Model file for the job. Use its own axes, mm. A direction names the side the tool comes from. Round coordinates to 2 decimals unless told otherwise and drop trailing zeros. Loops run counter-clockwise (first coordinate to the right, second up) from the corner with the lowest first, then second, coordinate; pieces in that order, holes last. Notation, with made-up numbers: M 78,15 L 137,15 A19 ccw 137,48 Z; hole C -17.5,-13 d11. An arc over 180 degrees is marked long. Use a Markdown table: item, result. Add a question column.
Item 1: Saw through at B-B on y = -10. Write the cut outline in (x, z).
Item 2: Saw through at D-D on z = 28. Write the cut outline in (x, y), then the cut area to 3 significant figures.
Item 3: Two-plate mould, pull along X, no slides. Class faces 1 (the flat face through (-2, -6, -35)), 2 (the flat face through (-10, -12.5, 8)), 3 (the cylindrical face through (-1.73, 7.81, -28.92)): +X half, -X half, draft (parallel to the pull), parting line (faces both ways), or undercut.
Item 4: Pin check, flat tips, straight feed: P1, Ø13, axis at x = -13.5, z = 17, coming from the -Y side; P2, Ø10, axis at y = -4, z = -30, coming from the -X side; P3, Ø1, axis at y = -7, z = -27, coming from the +X side; P4, Ø2, axis at y = -6, z = -30, coming from the -X side (3 decimals). Stop position of each tip, or through.
Item 5: Saw through at A-A on z = 0. Write the cut outline in (x, y).
Item 6: Wall check: L1, parallel to X at y = -4.25, z = 0; L2, parallel to Y at x = 14.5, z = 19; L3, parallel to Z at x = -20, y = -0.5. Give the ranges that are in metal, low to high. Write a range as from..to.
Item 7: Tool access for faces 4 (the cylindrical face through (6, 0, -40)), 5 (the flat face through (-19, -11, -19)), 6 (the flat face through (-19, 11, 18)): list every direction of +Z, -Z, +X, -X, +Y, -Y with a clear straight run to the whole face (end or side of a thin tool).
Item 8: Saw through at C-C on y = 0. Write the cut outline in (x, z), then the cut area to 3 significant figures.
```python
from build123d import *

# Parameters (mm, degrees)
SKETCH1_W           = 46
SKETCH1_H           = 46
BOSS_EXTRUDE1_DEPTH = 11
SKETCH2_R           = 19
BOSS_EXTRUDE2_DEPTH = 4.5
FILLET1_R           = 5
SKETCH3_R           = 16
CUT_EXTRUDE1_DEPTH  = 3
SKETCH4_R           = 12.5
CUT_EXTRUDE2_DEPTH  = 41.127920628
MIRROR1_START       = -12.5
MIRROR1_OUTLINE_R   = 16
MIRROR1_DEPTH       = 23.5
MIRROR1_START_2     = -15.5
MIRROR1_2_OUTLINE_W = 46
MIRROR1_2_OUTLINE_H = 46
MIRROR1_2_OUTLINE_R = 16
MIRROR1_2_DEPTH     = 4.5
SKETCH5_R           = 12.5
CUT_EXTRUDE3_DEPTH  = 42.955333564
SKETCH6_R           = 8
BOSS_EXTRUDE3_DEPTH = 12
SKETCH7_R           = 6
BOSS_EXTRUDE4_DEPTH = 10


with BuildPart() as part:
    # Sketch1 → Boss-Extrude1 (new, symmetric)
    with BuildSketch(Plane(origin=(0, 0, 0), x_dir=(1, 0, 0), z_dir=(0, 1, 0))):
        Rectangle(SKETCH1_W, SKETCH1_H)
    extrude(amount=BOSS_EXTRUDE1_DEPTH, both=True)

    # Sketch2 → Boss-Extrude2 (add)
    with BuildSketch(Plane(origin=(0, 11, 0), x_dir=(1, 0, 0), z_dir=(0, 1, 0))):
        with Locations(Location((0, 0, 0), (0, 0, 270))):
            Circle(SKETCH2_R)
    extrude(amount=BOSS_EXTRUDE2_DEPTH)

    # Fillet1
    # the kernel refuses this fillet: 5 mm, written as the material it adds along each edge
    with BuildSketch(Plane(origin=(0, 11, 0), x_dir=(0, 0, 1), z_dir=(-1, 0, 0))) as fillet1_piece_1_section:
        with BuildLine():
            CenterArc((23.974937186, 5), FILLET1_R, 185.739170477, 84.260829523)
            Line((19, 4.5), (19, 0))
            Line((19, 0), (23.974937186, 0))
        make_face()
    fillet1_piece_1 = revolve(axis=Axis((0, 11, 0), (0, 1, 0)), mode=Mode.PRIVATE)
    fillet1_piece_1 = split(fillet1_piece_1, bisect_by=Plane(origin=(0, 11, 23), z_dir=(0, 0, -1)), keep=Keep.TOP, mode=Mode.PRIVATE)
    fillet1_piece_1 = split(fillet1_piece_1, bisect_by=Plane(origin=(23, 11, 0), z_dir=(-1, 0, 0)), keep=Keep.TOP, mode=Mode.PRIVATE)
    fillet1_piece_1 = split(fillet1_piece_1, bisect_by=Plane(origin=(-23, 11, 0), z_dir=(1, 0, 0)), keep=Keep.TOP, mode=Mode.PRIVATE)
    fillet1_piece_1 = split(fillet1_piece_1, bisect_by=Plane(origin=(0, 11, -23), z_dir=(0, 0, 1)), keep=Keep.TOP, mode=Mode.PRIVATE)
    add(fillet1_piece_1)

    # Sketch3 → Cut-Extrude1 (cut)
    with BuildSketch(Plane(origin=(0, 15.5, 0), x_dir=(1, 0, 0), z_dir=(0, 1, 0))):
        with Locations(Location((0, 0, 0), (0, 0, 270))):
            Circle(SKETCH3_R)
    extrude(amount=-CUT_EXTRUDE1_DEPTH, mode=Mode.SUBTRACT)

    # Sketch4 → Cut-Extrude2 (cut, through all)
    with BuildSketch(Plane(origin=(0, 12.5, 0), x_dir=(1, 0, 0), z_dir=(0, 1, 0))):
        with Locations(Location((0, 0, 0), (0, 0, 270))):
            Circle(SKETCH4_R)
    extrude(amount=-CUT_EXTRUDE2_DEPTH, mode=Mode.SUBTRACT)

    # Mirror1: read off the stored shape, not the designer's step
    # Mirror1 outline → Mirror1 (add)
    with BuildSketch(Plane(origin=(0, 0, 0), x_dir=(1, 0, 0), z_dir=(0, 1, 0)).offset(MIRROR1_START)):
        Circle(MIRROR1_OUTLINE_R)
    extrude(amount=MIRROR1_DEPTH)

    # Mirror1 2 outline → Mirror1 2 (add)
    with BuildSketch(Plane(origin=(0, 0, 0), x_dir=(1, 0, 0), z_dir=(0, 1, 0)).offset(MIRROR1_START_2)):
        Rectangle(MIRROR1_2_OUTLINE_W, MIRROR1_2_OUTLINE_H)
        Circle(MIRROR1_2_OUTLINE_R, mode=Mode.SUBTRACT)
    extrude(amount=MIRROR1_2_DEPTH)

    # Mirror1 3 outline → Mirror1 3 (revolve, cut)
    with BuildSketch(Plane.XY):
        with BuildLine():
            Line((32.526911935, -11), (23.974937186, -11))
            ThreePointArc((23.974937186, -11), (20.620835219, -12.291900756), (19, -15.5))
            Line((19, -15.5), (32.526911935, -15.5))
            Line((32.526911935, -15.5), (32.526911935, -11))
        make_face()
    revolve(axis=Axis((0, 0, 0), (0, 1, 0)), mode=Mode.SUBTRACT)

    # Sketch5 → Cut-Extrude3 (cut, through all)
    with BuildSketch(Plane(origin=(0, 11, 0), x_dir=(1, 0, 0), z_dir=(0, 1, 0))):
        with Locations(Location((0, 0, 0), (0, 0, 270))):
            Circle(SKETCH5_R)
    extrude(amount=-CUT_EXTRUDE3_DEPTH, mode=Mode.SUBTRACT)

    # Sketch6 → Boss-Extrude3 (add)
    with BuildSketch(Plane(origin=(0, 0, -23), x_dir=(-1, 0, 0), z_dir=(0, 0, -1))):
        with Locations(Location((0, 0, 0), (0, 0, 180))):
            Circle(SKETCH6_R)
    boss_extrude3 = extrude(amount=BOSS_EXTRUDE3_DEPTH)

    # Sketch7 → Boss-Extrude4 (add)
    with BuildSketch(Plane(origin=(0, 0, -35), x_dir=(-1, 0, 0), z_dir=(0, 0, -1))):
        Circle(SKETCH7_R)
    boss_extrude4 = extrude(amount=BOSS_EXTRUDE4_DEPTH)

    # Mirror2: Boss-Extrude3, Boss-Extrude4 across plane
    add(boss_extrude3.mirror(Plane.XY))
    add(boss_extrude4.mirror(Plane.XY))


solid = part.part
```
Entries:
| question | item | result |
|---|---|---|
| 1 | outline | M -23,-23 L 23,-23 L 23,23 L -23,23 Z; hole C 0,0 d25 |
| 2 | outline | C 0,0 d16 |
| 2 | area | 201 mm2 |
| 3 | face 1 | draft |
| 3 | face 2 | undercut |
| 3 | face 3 | parting line |
| 4 | P1 | y = -15.5 |
| 4 | P2 | x = -8 |
| 4 | P3 | x = 4.66 |
| 4 | P4 | x = -6.245 |
| 5 | outline | M -23,-11.1 A5 cw -19,-15.5 L -16,-15.5 L -16,-12.5 L -12.5,-12.5 L -12.5,12.5 L -16,12.5 L -16,15.5 L -19,15.5 A5 cw -23,11.1 Z; M 12.5,-12.5 L 16,-12.5 L 16,-15.5 L 19,-15.5 A5 cw 23,-11.1 L 23,11.1 A5 cw 19,15.5 L 16,15.5 L 16,12.5 L 12.5,12.5 Z |
| 6 | L1 | -23..-12.5, 12.5..23 |
| 6 | L2 | -11..11 |
| 6 | L3 | -23..23 |
| 7 | face 4 | -Z |
| 7 | face 5 | -Z, -X, -Y |
| 7 | face 6 | +Z, -X, +Y |
| 8 | outline | M -23,-23 L -8,-23 L -8,-35 L -6,-35 L -6,-45 L 6,-45 L 6,-35 L 8,-35 L 8,-23 L 23,-23 L 23,23 L 8,23 L 8,35 L 6,35 L 6,45 L -6,45 L -6,35 L -8,35 L -8,23 L -23,23 Z; hole C 0,0 d25 |
| 8 | area | 2,250 mm2 |
